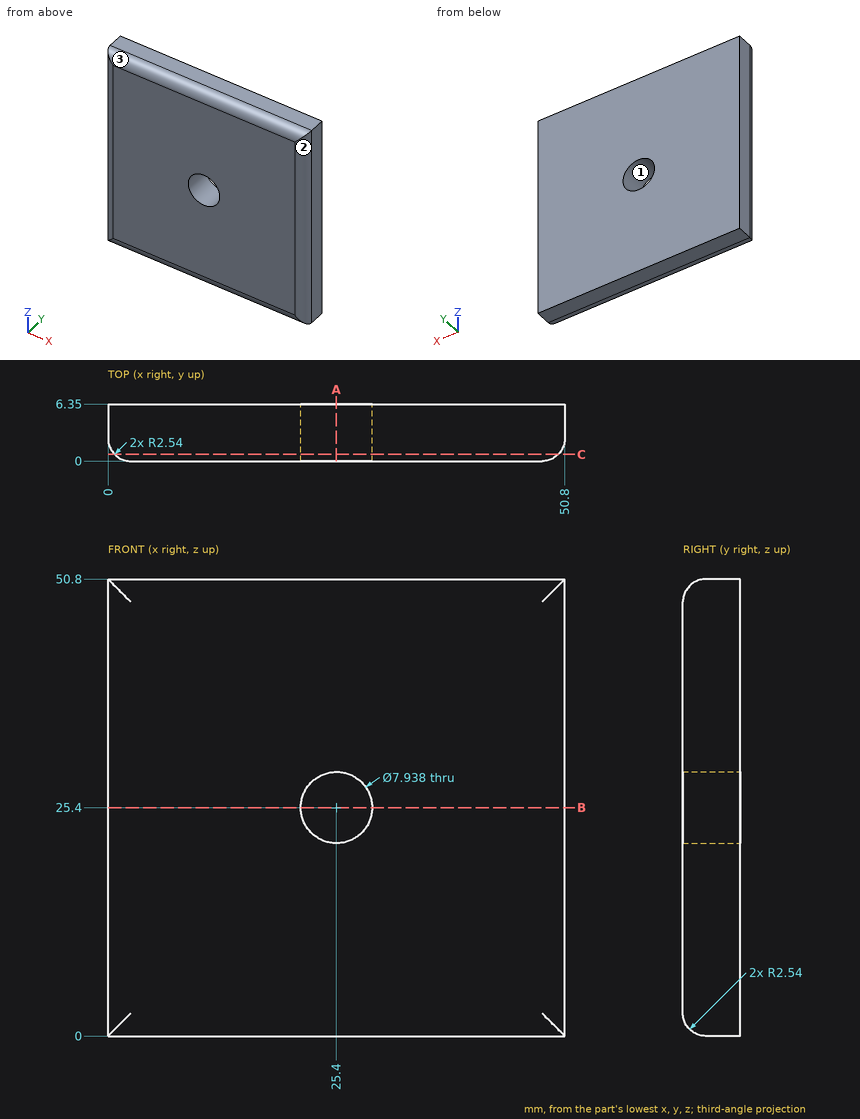
Geometry: see drawing. Coordinates: mm, zero at the bounding-box minimum. Coordinates: 2 decimals unless noted, no trailing zeros. Order: outer loops, then holes, each group sorted by start corner. A loop starts at its lowest first (then second) coordinate and runs counter-clockwise, first axis right, second up. Notation, with made-up numbers: M 63.5,81 L 76.5,81 A20 cw 76.5,109 Z; hole C 75.25,65.5 d9. An arc over 180 degrees is marked long. Answer in a Markdown table with one row per item. Add a question column.
Q1. Section query B-B on z = 25.4. Return the cut outline in (x, y).
Q2. Section query C-C on y = 0.75. Return the cut outline in (x, z), and give its area (3 significant figures).
Q3. Mould query, pull axis X, two halves, no side actions, for the marked faces 1, 2 and 3. Classes: released by +X, released by -X, zero draft, split by the parting line, or undercut.
Q4. Contact query for a flat-ended pin moving along its axis: P1, Ø10.5, axis at x = 25.4, z = 25.4, coming from the +Y side. Output: stop coordinate, or through.
Q5. Section query A-A on x = 25.4. Return the cut outline in (y, z).
Q6. Line query: L1, parallel to Z at x = 25.5, y = 5.25; L2, parallel to Z at x = 28.5, y = 6 (1 decimal); L3, parallel to X at y = 1, z = 23. Output: solid intervals per line, ascending.
Completed:
| question | item | result |
|---|---|---|
| 1 | outline | M 0,2.54 A2.54 ccw 2.54,0 L 21.43,0 L 21.43,6.35 L 0,6.35 Z; M 29.37,0 L 48.26,0 A2.54 ccw 50.8,2.54 L 50.8,6.35 L 29.37,6.35 Z |
| 2 | outline | M 0.74,0.74 L 50.06,0.74 L 50.06,50.06 L 0.74,50.06 Z; hole C 25.4,25.4 d7.94 |
| 2 | area | 2,380 mm2 |
| 3 | face 1 | undercut |
| 3 | face 2 | released by +X |
| 3 | face 3 | zero draft |
| 4 | P1 | stops at y = 6.35 |
| 5 | outline | M 0,2.54 A2.54 ccw 2.54,0 L 6.35,0 L 6.35,21.43 L 0,21.43 Z; M 0,29.37 L 6.35,29.37 L 6.35,50.8 L 2.54,50.8 A2.54 ccw 0,48.26 Z |
| 6 | L1 | z = 0 to 21.43, 29.37 to 50.8 |
| 6 | L2 | z = 0 to 22.9, 27.9 to 50.8 |
| 6 | L3 | x = 0.52 to 22.24, 28.56 to 50.28 |
